Work out the finished part from the listing and answer in its coordinate system (mm). Face numbers are marked on the shaded views. Round coordinates to 2 decimals unless told otherwise and drop trailing zeros. Order: outer loops, then holes, each group sorted by start corner. A loop starts at its lowest first (then second) coordinate and runs counter-clockwise, first axis right, second up. Notation, with made-up numbers: (-7, -20.75) - (26, -20.75) arc R12 cw to (26, -8.75) - close; hole circle Ø6 at (54.25, -26.75). An arc over 180 degrees is marked (long way). One line per question, with ' | ' between items. Start each with the question number.
from build123d import *

# Parameters (mm, degrees)
BOSS_EXTRUDE1_DEPTH      = 406.4
BOSS_EXTRUDE1_DEPTH_BACK = 3.175
SKETCH1_W                = 50.8
SKETCH1_H                = 50.8
SKETCH1_W_2              = 44.45
SKETCH1_H_2              = 44.45
SKETCH1_3_W              = 44.45
SKETCH1_3_H              = 44.45
SKETCH1_3_W_2            = 25.4
SKETCH1_3_H_2            = 25.4
BOSS_EXTRUDE2_DEPTH      = 3.175
SKETCH1_4_W              = 25.4
SKETCH1_4_H              = 25.4
BOSS_EXTRUDE3_DEPTH      = 3.175
CUT_EXTRUDE3_REACH       = 414.701
SKETCH4_R                = 1.5875
SKETCH4_R_2              = 1.651
SKETCH4_W                = 31.75
SKETCH4_H                = 127
CUT_EXTRUDE4_REACH       = 414.701
SKETCH5_R                = 1.5875
SKETCH5_R_2              = 6.35
FILLET1_R                = 2.54
FILLET4_R                = 2.54
SKETCH7_W                = 407.035
SKETCH7_H                = 3.175
BOSS_EXTRUDE4_DEPTH      = 6.35
FILLET5_R                = 1.5875


with BuildPart() as part:
    # Sketch1 → Boss-Extrude1 (new, two sides: drawn at the far end of the back side and taken through both)
    with BuildSketch(Plane.XY.offset(-BOSS_EXTRUDE1_DEPTH_BACK)):
        with Locations((25.4, 25.4)):
            Rectangle(SKETCH1_W, SKETCH1_H)
        with Locations((25.4, 25.4)):
            Rectangle(SKETCH1_W_2, SKETCH1_H_2, mode=Mode.SUBTRACT)
    extrude(amount=BOSS_EXTRUDE1_DEPTH + BOSS_EXTRUDE1_DEPTH_BACK)

    # Sketch1<3> → Boss-Extrude2 (add)
    with BuildSketch(Plane.XY):
        with Locations((25.4, 25.4)):
            Rectangle(SKETCH1_3_W, SKETCH1_3_H)
        with Locations((25.4, 25.4)):
            Rectangle(SKETCH1_3_W_2, SKETCH1_3_H_2, mode=Mode.SUBTRACT)
    extrude(amount=-BOSS_EXTRUDE2_DEPTH)

    # Sketch1<4> → Boss-Extrude3 (add)
    with BuildSketch(Plane.XY):
        with Locations((25.4, 25.4)):
            Rectangle(SKETCH1_4_W, SKETCH1_4_H)
    extrude(amount=-BOSS_EXTRUDE3_DEPTH)

    # Cut-Extrude3: up to this face of the body (flat: up to its plane)
    cut_extrude3_end = Plane(part.part.faces().sort_by_distance((25.4, 0, 201.6125))[0])
    # Sketch4 → Cut-Extrude3 (cut, up to the picked face)
    with BuildSketch(Plane(origin=(0, 50.8, 0), x_dir=(1, 0, 0), z_dir=(0, 1, 0)), mode=Mode.PRIVATE) as cut_extrude3_sk1:
        with Locations(Location((25.4, -381, 0), (0, 0, 270))):
            Circle(SKETCH4_R)
    cut_extrude3_tool1 = split(extrude(cut_extrude3_sk1.sketch, amount=-CUT_EXTRUDE3_REACH, mode=Mode.PRIVATE), bisect_by=cut_extrude3_end, keep=Keep.BOTH, mode=Mode.PRIVATE)
    # Sketch4 → Cut-Extrude3 (cut, up to the picked face)
    with BuildSketch(Plane(origin=(0, 50.8, 0), x_dir=(1, 0, 0), z_dir=(0, 1, 0)), mode=Mode.PRIVATE) as cut_extrude3_sk2:
        with Locations(Location((25.4, -28.575, 0), (0, 0, 270))):
            Circle(SKETCH4_R_2)
    cut_extrude3_tool2 = split(extrude(cut_extrude3_sk2.sketch, amount=-CUT_EXTRUDE3_REACH, mode=Mode.PRIVATE), bisect_by=cut_extrude3_end, keep=Keep.BOTH, mode=Mode.PRIVATE)
    # Sketch4 → Cut-Extrude3 (cut, up to the picked face)
    with BuildSketch(Plane(origin=(0, 50.8, 0), x_dir=(1, 0, 0), z_dir=(0, 1, 0)), mode=Mode.PRIVATE) as cut_extrude3_sk3:
        with Locations((25.4, -177.8)):
            Rectangle(SKETCH4_W, SKETCH4_H)
    cut_extrude3_tool3 = split(extrude(cut_extrude3_sk3.sketch, amount=-CUT_EXTRUDE3_REACH, mode=Mode.PRIVATE), bisect_by=cut_extrude3_end, keep=Keep.BOTH, mode=Mode.PRIVATE)
    add(cut_extrude3_tool1.solids().sort_by(Axis((25.4, 50.8, 381), (0, -1, 0)))[0], mode=Mode.SUBTRACT)
    add(cut_extrude3_tool2.solids().sort_by(Axis((25.4, 50.8, 28.575), (0, -1, 0)))[0], mode=Mode.SUBTRACT)
    add(cut_extrude3_tool3.solids().sort_by(Axis((25.4, 50.8, 177.8), (0, -1, 0)))[0], mode=Mode.SUBTRACT)

    # Cut-Extrude4: up to this face of the body (flat: up to its plane)
    cut_extrude4_end = Plane(part.part.faces().sort_by_distance((0, 25.4, 201.6125))[0])
    # Sketch5 → Cut-Extrude4 (cut, up to the picked face)
    with BuildSketch(Plane(origin=(50.8, 0, 0), x_dir=(0, 0, -1), z_dir=(1, 0, 0)), mode=Mode.PRIVATE) as cut_extrude4_sk1:
        with Locations((-381, 25.4)):
            Circle(SKETCH5_R)
    cut_extrude4_tool1 = split(extrude(cut_extrude4_sk1.sketch, amount=-CUT_EXTRUDE4_REACH, mode=Mode.PRIVATE), bisect_by=cut_extrude4_end, keep=Keep.BOTH, mode=Mode.PRIVATE)
    # Sketch5 → Cut-Extrude4 (cut, up to the picked face)
    with BuildSketch(Plane(origin=(50.8, 0, 0), x_dir=(0, 0, -1), z_dir=(1, 0, 0)), mode=Mode.PRIVATE) as cut_extrude4_sk2:
        with Locations((-177.8, 25.4)):
            Circle(SKETCH5_R_2)
    cut_extrude4_tool2 = split(extrude(cut_extrude4_sk2.sketch, amount=-CUT_EXTRUDE4_REACH, mode=Mode.PRIVATE), bisect_by=cut_extrude4_end, keep=Keep.BOTH, mode=Mode.PRIVATE)
    add(cut_extrude4_tool1.solids().sort_by(Axis((50.8, 25.4, 381), (-1, 0, 0)))[0], mode=Mode.SUBTRACT)
    add(cut_extrude4_tool2.solids().sort_by(Axis((50.8, 25.4, 177.8), (-1, 0, 0)))[0], mode=Mode.SUBTRACT)

    # Fillet1
    fillet1_edges = [part.edges().sort_by_distance(p)[0] for p in [
        (0, 0, 201.6125),
        (0, 50.8, 201.6125),
        (50.8, 50.8, 201.6125),
        (50.8, 0, 201.6125),
        (25.4, 0, -3.175),
        (50.8, 25.4, -3.175),
        (25.4, 50.8, -3.175),
        (0, 25.4, -3.175),
    ]]
    fillet(fillet1_edges, radius=FILLET1_R)

    # Fillet4
    fillet4_edges = [part.edges().sort_by_distance(p)[0] for p in [
        (3.175, 47.625, 203.2),
        (3.175, 3.175, 203.2),
        (47.625, 47.625, 203.2),
        (47.625, 3.175, 203.2),
    ]]
    fillet(fillet4_edges, radius=FILLET4_R)

    # Sketch7 → Boss-Extrude4 (add)
    with BuildSketch(Plane(origin=(50.8, 0, 0), x_dir=(0, 0, -1), z_dir=(1, 0, 0))):
        with Locations((-202.8825, 46.6725)):
            Rectangle(SKETCH7_W, SKETCH7_H)
        with Locations((-202.8825, 4.1275)):
            Rectangle(SKETCH7_W, SKETCH7_H)
    extrude(amount=BOSS_EXTRUDE4_DEPTH)

    # Fillet5
    fillet5_edges = [part.edges().sort_by_distance(p)[0] for p in [
        (9.525, 1.5875, 114.3),
        (9.525, 1.5875, 241.3),
        (41.275, 1.5875, 241.3),
        (41.275, 1.5875, 114.3),
        (9.525, 49.2125, 114.3),
        (9.525, 49.2125, 241.3),
        (41.275, 49.2125, 241.3),
        (41.275, 49.2125, 114.3),
    ]]
    fillet(fillet5_edges, radius=FILLET5_R)


solid = part.part
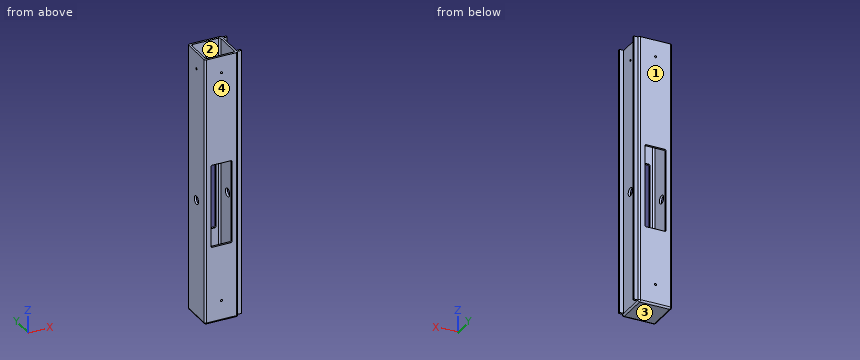
1) Determine the mould class of the marked faces 1, 2, 3 and 4 for opening direction Y: released by +Y, released by -Y, zero draft, split by the parting line, or undercut.
2) Section D-D on z = 177.8 is taken. Give the number of separate pieces and of enclosed holes in the cut face, and give its area (3 significant figures).
3) Straight lines are drawn through the part: line 1 (X direction, y = 20, z = 131.5) (3 decimals); line 2 (Z direction, x = 25, y = 2). For each, find the intervals that lie inside material, in ascending order.
4) Flat-ended cylindrical pins translate along their axes: pin 1 (1 mm diameter, centred on x = 26, y = 1.5, fed in from -Z); pin 2 (22 mm diameter, centred on x = 27.5, y = 27, fed in from +Z); pin 3 (7 mm diameter, centred on x = 55, z = 303.5, fed in from -Y). Find the tip coordinate at first contact, or state that the pin passes through.
5) Section A-A on x = 31 is taken. Give the vertices of the cut face in (y, z) (3 decimals), and give its area (3 significant figures).
6) Section C-C on z = 311.5 is taken. Give the vertices of the cut face in (x, y) (3 decimals), and give its area (3 significant figures).
Recorded:
1) face 1: released by +Y | face 2: undercut | face 3: zero draft | face 4: released by -Y
2) separate pieces: 4 | enclosed holes: 0 | area: 363 mm²
3) line 1: x = 0 to 3.175, 47.625 to 50.8 | line 2: z = -3.12 to 26.97, 30.18 to 114.3, 241.3 to 379.46, 382.54 to 406.4
4) pin 1: stops at z = -3.12 | pin 2: stops at z = 0 | pin 3: stops at y = 2.54
5) outline: (0, -0.635) arc R2.54 ccw to (2.54, -3.175) - (48.26, -3.175) arc R2.54 ccw to (50.8, -0.635) - (50.8, 114.3) - (47.625, 114.3) - (47.625, 0) - (3.175, 0) - (3.175, 114.3) - (0, 114.3) - close; (0, 241.3) - (3.175, 241.3) - (3.175, 406.4) - (0, 406.4) - close; (47.625, 241.3) - (50.8, 241.3) - (50.8, 406.4) - (47.625, 406.4) - close | area: 1,930 mm²
6) outline: (0, 2.54) arc R2.54 ccw to (2.54, 0) - (48.26, 0) arc R2.54 ccw to (50.8, 2.54) - (57.15, 2.54) - (57.15, 5.715) - (50.8, 5.715) - (50.8, 45.085) - (57.15, 45.085) - (57.15, 48.26) - (50.8, 48.26) arc R2.54 ccw to (48.26, 50.8) - (2.54, 50.8) arc R2.54 ccw to (0, 48.26) - close; hole (3.175, 5.715) arc R2.54 ccw to (5.715, 3.175) - (45.085, 3.175) arc R2.54 ccw to (47.625, 5.715) - (47.625, 45.085) arc R2.54 ccw to (45.085, 47.625) - (5.715, 47.625) arc R2.54 ccw to (3.175, 45.085) - close | area: 645 mm²
